from build123d import *

# Parameters (mm, degrees)
BOSS_EXTRUDE1_DEPTH = 64.2
SKETCH2_R           = 1.5
CUT_EXTRUDE1_DEPTH  = 5


with BuildPart() as part:
    # Sketch1 → Boss-Extrude1 (new body)
    with BuildSketch(Plane.XY):
        Polygon((0, 0), (0, 41), (3.95, 41), (3.95, 31), (10.3, 31), (10.3, 9), (8.55, 9), (8.55, 4), (13, 4), (13, 0), align=None)
    extrude(amount=BOSS_EXTRUDE1_DEPTH)

    # Sketch2 → Cut-Extrude1 (cut)
    with BuildSketch(Plane.XY.offset(64.2)):
        with Locations((3, 28)):
            Circle(SKETCH2_R)
        with Locations((3, 10)):
            Circle(SKETCH2_R)
    cut_extrude1 = extrude(amount=-CUT_EXTRUDE1_DEPTH, mode=Mode.SUBTRACT)

    # Mirror1: Cut-Extrude1 across plane
    add(cut_extrude1.mirror(Plane.XY.offset(32.1)), mode=Mode.SUBTRACT)


solid = part.part
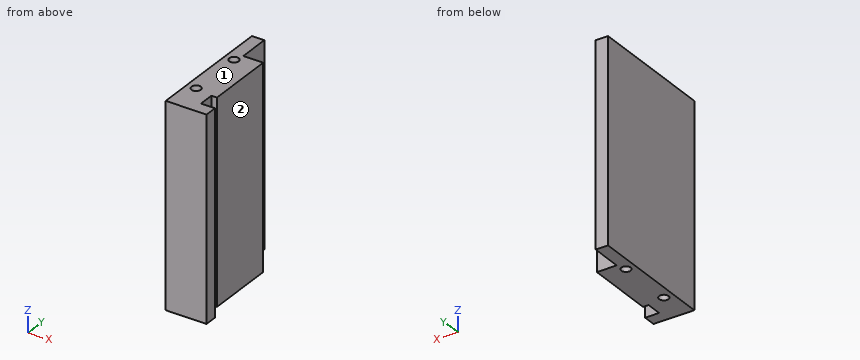
Design review of the part built by this model. Coordinates are the model's own, in mm. Face numbers are marked on the shaded views. A direction names the side the tool comes from. Coordinates: 2 decimals unless noted, no trailing zeros. Loops run counter-clockwise (first coordinate to the right, second up) from the corner with the lowest first, then second, coordinate; pieces in that order, holes last.
Item 1: Add section D-D (y = 33.5). Write out the cut boundary in (x, z).
Completed:
outline: (0, 0) - (3.95, 0) - (3.95, 64.2) - (0, 64.2) - close
Item 2: For the marked faces 1 and 2, list the 3-axis set-ups (+Z, -Z, +X, -X, +Y, -Y) from which the entire face can be reached by the end or side of a thin tool; tool diameter is ignored.
Completed:
face 1: +Z, +X, -X, +Y, -Y
face 2: +Z, -Z, +X, +Y
Item 3: Add section C-C (y = 28). Write out the cut boundary in (x, z).
Completed:
outline: (0, 0) - (1.5, 0) - (1.5, 5) - (4.5, 5) - (4.5, 0) - (10.3, 0) - (10.3, 64.2) - (4.5, 64.2) - (4.5, 59.2) - (1.5, 59.2) - (1.5, 64.2) - (0, 64.2) - close
Item 4: Add section A-A (x = 3). Write out the cut boundary in (y, z).
Completed:
outline: (0, 0) - (8.5, 0) - (8.5, 5) - (11.5, 5) - (11.5, 0) - (26.5, 0) - (26.5, 5) - (29.5, 5) - (29.5, 0) - (41, 0) - (41, 64.2) - (29.5, 64.2) - (29.5, 59.2) - (26.5, 59.2) - (26.5, 64.2) - (11.5, 64.2) - (11.5, 59.2) - (8.5, 59.2) - (8.5, 64.2) - (0, 64.2) - close
Item 5: Add section B-B (z = 15.5). Write out the cut boundary in (x, y).
Completed:
outline: (0, 0) - (13, 0) - (13, 4) - (8.55, 4) - (8.55, 9) - (10.3, 9) - (10.3, 31) - (3.95, 31) - (3.95, 41) - (0, 41) - close
Item 6: Clearance check with flat-ended pins moving along their axes: pin 1 (24 mm diameter, centred on y = 17, z = 37.5, fed in from +X); pin 2 (3 mm diameter, centred on y = 35, z = 37.5, fed in from +X); pin 3 (2.5 mm diameter, centred on x = 3, y = 28, fed in from -Z). State where each tip first meets the part, or that it passes through.
Completed:
pin 1: stops at x = 10.3
pin 2: stops at x = 3.95
pin 3: stops at z = 5
Item 7: Wall thickness on L1, parallel to Y at x = 3, z = 60.45; L2, parallel to Y at x = 9, z = 55; L3, parallel to Y at x = 12.75, z = 8: over which ranges is each line inside the solid? List them lowest first.
Completed:
L1: y = 0 to 8.5, 11.5 to 26.5, 29.5 to 41
L2: y = 0 to 4, 9 to 31
L3: y = 0 to 4
